Input: part model. Units: mm. Frame: model coordinates. A direction names the side the tool comes from. Give positions to 0.01 mm unless a question says otherwise; leave off trailing zeros.
```python
from build123d import *

# Parameters (mm, degrees)
SKETCH1_W           = 482.6
SKETCH1_H           = 101.6
BOSS_EXTRUDE1_DEPTH = 12.7
SKETCH2_R           = 2.7813
CUT_EXTRUDE1_DEPTH  = 13.7
SKETCH3_R           = 1.5875
CUT_EXTRUDE2_DEPTH  = 13.7
SKETCH4_R           = 0.79375
CUT_EXTRUDE3_DEPTH  = 13.7
SKETCH5_R           = 0.79375
CUT_EXTRUDE4_DEPTH  = 13.7
CUT_EXTRUDE5_DEPTH  = 13.7


with BuildPart() as part:
    # Sketch1 → Boss-Extrude1 (new body)
    with BuildSketch(Plane(origin=(0, 0, 0), x_dir=(1, 0, 0), z_dir=(0, 1, 0))):
        Rectangle(SKETCH1_W, SKETCH1_H)
    extrude(amount=BOSS_EXTRUDE1_DEPTH)

    # Sketch2 → Cut-Extrude1 (cut, through all)
    with BuildSketch(Plane(origin=(0, 12.7, 0), x_dir=(1, 0, 0), z_dir=(0, 1, 0))):
        with Locations((-232.5624, 38.1)):
            Circle(SKETCH2_R)
        with Locations((-232.5624, -38.1)):
            Circle(SKETCH2_R)
        with Locations((232.5624, 38.1)):
            Circle(SKETCH2_R)
        with Locations((232.5624, -38.1)):
            Circle(SKETCH2_R)
    extrude(amount=-CUT_EXTRUDE1_DEPTH, mode=Mode.SUBTRACT)

    # Sketch3 → Cut-Extrude2 (cut, through all)
    with BuildSketch(Plane(origin=(0, 12.7, 0), x_dir=(1, 0, 0), z_dir=(0, 1, 0))):
        with Locations((-25.4, 25.4)):
            Circle(SKETCH3_R)
        with Locations((25.4, 25.4)):
            Circle(SKETCH3_R)
        with Locations((25.4, -25.4)):
            Circle(SKETCH3_R)
        with Locations((-25.4, -25.4)):
            Circle(SKETCH3_R)
    extrude(amount=-CUT_EXTRUDE2_DEPTH, mode=Mode.SUBTRACT)

    # Sketch4 → Cut-Extrude3 (cut, through all)
    with BuildSketch(Plane(origin=(0, 12.7, 0), x_dir=(1, 0, 0), z_dir=(0, 1, 0))):
        with Locations((-25.4, 0)):
            Circle(SKETCH4_R)
        with Locations((25.4, 0)):
            Circle(SKETCH4_R)
        with Locations((-50.8, 0)):
            Circle(SKETCH4_R)
        with Locations((50.8, 0)):
            Circle(SKETCH4_R)
        with Locations((-107.95, 12.7)):
            Circle(SKETCH4_R)
        with Locations((-107.95, -12.7)):
            Circle(SKETCH4_R)
        with Locations((107.95, -12.7)):
            Circle(SKETCH4_R)
        with Locations((107.95, 12.7)):
            Circle(SKETCH4_R)
    extrude(amount=-CUT_EXTRUDE3_DEPTH, mode=Mode.SUBTRACT)

    # Sketch5 → Cut-Extrude4 (cut, through all)
    with BuildSketch(Plane(origin=(0, 12.7, 0), x_dir=(1, 0, 0), z_dir=(0, 1, 0))):
        with Locations((95.25, 0)):
            Circle(SKETCH5_R)
        with Locations((120.65, 0)):
            Circle(SKETCH5_R)
    extrude(amount=-CUT_EXTRUDE4_DEPTH, mode=Mode.SUBTRACT)

    # Sketch6 → Cut-Extrude5 (cut, through all)
    with BuildSketch(Plane(origin=(0, 12.7, 0), x_dir=(1, 0, 0), z_dir=(0, 1, 0))):
        with BuildLine():
            Line((125.489928348, -20.1549), (125.489928348, -29.3751))
            ThreePointArc((125.489928348, -29.3751), (127.864828348, -31.75), (130.239728348, -29.3751))
            Line((130.239728348, -29.3751), (130.239728348, -20.1549))
            ThreePointArc((130.239728348, -20.1549), (127.864828348, -17.78), (125.489928348, -20.1549))
        make_face()
    extrude(amount=-CUT_EXTRUDE5_DEPTH, mode=Mode.SUBTRACT)


solid = part.part
```
Item 1: Set-up query: faces 1 (the flat face through (125.49, 6, 25)), 2 (the flat face through (-3, 6, 50.8)). Return all of +Z, -Z, +X, -X, +Y, -Y with unobstructed straight access to the full face (end or side cutting, diameter ignored); none if empty.
Item 2: Pin query (flat end, axial travel): pin 1 (1.3 mm diameter, centred on x = -107.95, z = 12.7, fed in from +Y). Return the tip coordinate at first contact, or that it passes through.
Item 3: Mould query, pull axis X, two halves, no side actions, for faces 3 (the flat face through (241.3, 6, 1)), 4 (the flat face through (-241.3, 6, 1)), 5 (the flat face through (130.24, 6, 25)), 6 (the flat face through (-3, 12.7, -1)). Classes: +X half, -X half, draft (parallel to the pull), parting line (faces both ways), or undercut.
Item 4: Ray query, line 1 (X direction, y = 3.25, z = -12.7); line 2 (Z direction, x = -25.4, y = 7.25); line 3 (Z direction, x = -107.95, y = 7.75). Return the intervals inside material, ascending.
Solved:
1. face 1: +Y, -Y
1. face 2: +Z, +X, -X, +Y, -Y
2. pin 1: passes through
3. face 3: +X half
3. face 4: -X half
3. face 5: undercut
3. face 6: draft
4. line 1: x = -241.3 to -108.74, -107.16 to 107.16, 108.74 to 241.3
4. line 2: z = -50.8 to -26.99, -23.81 to -0.79, 0.79 to 23.81, 26.99 to 50.8
4. line 3: z = -50.8 to -13.49, -11.91 to 11.91, 13.49 to 50.8
